Read the model definition and answer for the solid it produces. Units are mm, in the model's axes. Coordinates: 2 decimals unless noted, no trailing zeros. Write each loop counter-clockwise with the first axis right and the second up, starting at its lowest first coordinate (ties: lowest second). Pieces come first, ordered by that corner, then holes. Notation, with made-up numbers: (2, -6) -> (39, -6) arc R22 cw to (39, 19) -> close; hole circle Ø5 at (-21, -1). An arc over 180 degrees is marked (long way). Write item = value, one per line. Start each with the question number.
1) Section A-A (y = -0.75) is taken. Determine the outline of the cut face in (x, z).
2) Flat-ended cylindrical pins translate along their axes: pin 1 Ø3 at (y, z) = (-2, -8.5) entering from +X; pin 2 Ø1.5 at (x, y) = (9.5, -2.5) entering from -Z; pin 3 Ø4 at (x, y) = (-17, 1) entering from +Z. Find the tip coordinate at first contact, or state that the pin passes through.
3) Find the intervals of material crossed by line 1 along Y through (x, z) = (19.5, 4); line 2 along Z through (x, y) = (-4.5, 1.5); line 3 along Z through (x, y) = (6, -2), in increasing order. Write a range as from..to.
4) Section B-B (y = -3) is taken. Determine the outline of the cut face in (x, z), plus the area to 3 significant figures.
from build123d import *

# Parameters (mm, degrees)
F1_DEPTH = 3.81
F2_R     = 2.54


with BuildPart() as f1:
    # F0 (on Front) → F1 (new body, symmetric)
    with BuildSketch(Plane.XZ):
        with BuildLine():
            ThreePointArc((0, -22.272892), (15.749313, -15.749313), (22.272892, 0))
            ThreePointArc((22.272892, 0), (15.749313, 15.749313), (0, 22.272892))
            Line((0, 22.272892), (0, 13.651826))
            ThreePointArc((0, 13.651826), (9.653299, 9.653299), (13.651826, 0))
            ThreePointArc((13.651826, 0), (9.653299, -9.653299), (0, -13.651826))
            Line((0, -13.651826), (0, -22.272892))
        make_face()
        with BuildLine():
            Line((0, 13.651826), (0, 22.272892))
            ThreePointArc((0, 22.272892), (-22.272892, 0), (0, -22.272892))
            Line((0, -22.272892), (0, -13.651826))
            ThreePointArc((0, -13.651826), (-13.651826, 0), (0, 13.651826))
        make_face()
    extrude(amount=F1_DEPTH, both=True)

    # F2
    f2_edges = [f1.edges().sort_by_distance(p)[0] for p in [
        (-13.651826, -3.81, 0),
        (-22.272892, -3.81, 0),
        (-22.272892, 3.81, 0),
        (-13.651826, 3.81, 0),
    ]]
    fillet(f2_edges, radius=F2_R)


solid = f1.part
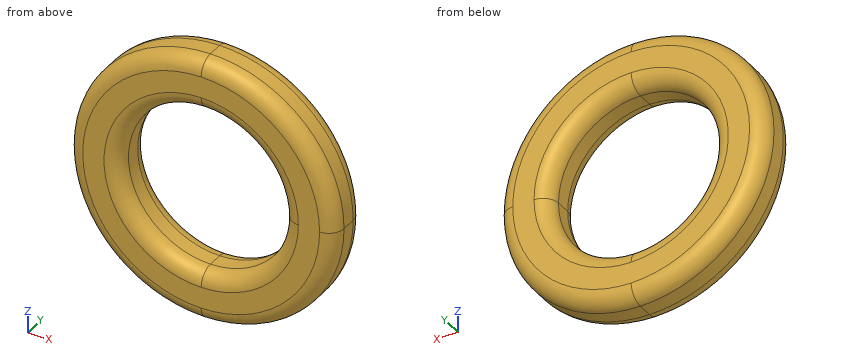
Answer key:
q1.outline = circle Ø44.55 at (0, 0); hole (0, -13.65) arc R13.65 ccw to (13.65, 0) arc R13.65 ccw (long way) to start
q2.pin_1 = 21.11
q2.pin_2 = -20.28
q2.pin_3 = 16.46
q3.line_1 = -3.8..3.8
q3.line_2 = -21.8..-12.9, 12.9..21.8
q3.line_3 = -21.34..-12.38, 12.38..21.34
q4.outline = circle Ø43.19 at (0, 0); hole (0, -14.33) arc R14.33 ccw to (14.33, 0) arc R14.33 ccw (long way) to start
q4.area = 819 mm^2
